Verification items for the finished model (mm, model axes). Face numbers are marked on the shaded views. A direction names the side the tool comes from. Round coordinates to 2 decimals unless told otherwise and drop trailing zeros. Order: outer loops, then holes, each group sorted by start corner. A loop starts at its lowest first (then second) coordinate and runs counter-clockwise, first axis right, second up. Notation, with made-up numbers: (51.25, -9) -> (73.25, -9) arc R21 ccw to (73.25, 5) -> close; hole circle Ø8 at (79, -30.5). An arc over 180 degrees is marked (long way). Return JSON: item names as keys, results as strings. Group by question number.
Item 1: Sectioned sample at D-D on z = 45.5. Record the cut outline in (x, y) (3 decimals), plus the area to 3 significant figures.
Item 2: Access from +Z, -Z, +X, -X, +Y, -Y to the whole of each face (thin tool, end or side, straight path). Record for the marked faces 4 and 5.
Item 3: Sectioned sample at A-A on x = 58.5. Record the cut outline in (y, z) (3 decimals), plus the area to 3 significant figures.
Item 4: Sectioned sample at C-C on y = 19. Record the cut outline in (x, z) (3 decimals).
Item 5: Sectioned sample at B-B on z = 27.5. Record the cut outline in (x, y) (3 decimals), plus the area to 3 significant figures.
Item 6: Draft check along Z on the marked faces 1, 2 and 3. Enter one of: pulls with the +Z half, pulls with the -Z half, needs draft (parallel to the pull), parting line crosses it, or undercut.
Item 7: Depth check by flat-ended pin: pin 1 Ø1 at (y, z) = (4.5, -1.5) entering from -X; pin 2 Ø1 at (y, z) = (6.5, -1) entering from +X; pin 3 Ø2 at (x, z) = (44.5, 22) entering from +Y. Enter the tip coordinate at first touch or a pass-through.
Item 8: Scan lines: probe 1 along Z at (x, y) = (33, 21) (3 decimals); probe 2 along X at (y, z) = (7.5, -1) (3 decimals); probe 3 along X at (y, z) = (34, 35.5) (3 decimals). Record each from-to range of solid material in increasing order. Write a range as from..to.
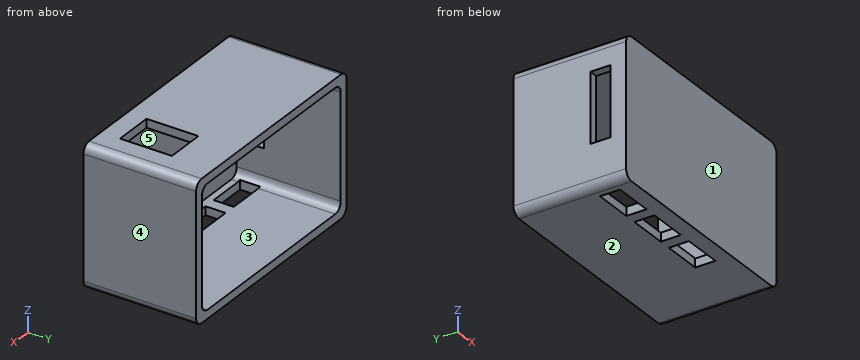
```python
from build123d import *

# Parameters (mm, degrees)
SKETCH1_W           = 76.2
SKETCH1_H           = 44.45
BOSS_EXTRUDE1_DEPTH = 38.1
SHELL1_T            = 3.175
SKETCH3_W           = 25.4
SKETCH3_H           = 7.366
CUT_EXTRUDE2_DEPTH  = 12.7
FILLET1_R           = 3.048
SKETCH6_W           = 14.605
SKETCH6_H           = 19.05
CUT_EXTRUDE4_DEPTH  = 12.7
SKETCH5_W           = 14.478
SKETCH5_H           = 7.366
CUT_EXTRUDE5_DEPTH  = 12.7


with BuildPart() as part:
    # Sketch1 → Boss-Extrude1 (new body)
    with BuildSketch(Plane(origin=(0, 0, 0), x_dir=(1, 0, 0), z_dir=(0, 1, 0))):
        with Locations((38.1, -22.225)):
            Rectangle(SKETCH1_W, SKETCH1_H)
    extrude(amount=BOSS_EXTRUDE1_DEPTH)

    # Shell1
    shell1_openings = [part.faces().sort_by_distance(p)[0] for p in [
        (38.1, 38.1, 22.225),
    ]]
    offset(amount=SHELL1_T, openings=shell1_openings, kind=Kind.INTERSECTION)

    # Sketch3 → Cut-Extrude2 (cut)
    with BuildSketch(Plane.ZY.offset(3.175)):
        with Locations((25.4, 6.223)):
            Rectangle(SKETCH3_W, SKETCH3_H)
    extrude(amount=-CUT_EXTRUDE2_DEPTH, mode=Mode.SUBTRACT)

    # Fillet1
    fillet1_edges = [part.edges().sort_by_distance(p)[0] for p in [
        (0, 19.05, 0),
        (0, 19.05, 44.45),
        (76.2, 19.05, 44.45),
        (76.2, 19.05, 0),
        (-3.175, 17.4625, -3.175),
        (79.375, 17.4625, -3.175),
        (79.375, 17.4625, 47.625),
        (-3.175, 17.4625, 47.625),
    ]]
    fillet(fillet1_edges, radius=FILLET1_R)

    # Sketch6 → Cut-Extrude4 (cut)
    with BuildSketch(Plane.XY.offset(47.625)):
        with Locations((62.5475, 13.335)):
            Rectangle(SKETCH6_W, SKETCH6_H)
    extrude(amount=-CUT_EXTRUDE4_DEPTH, mode=Mode.SUBTRACT)

    # Sketch5 → Cut-Extrude5 (cut)
    with BuildSketch(Plane(origin=(0, 0, -3.175), x_dir=(-1, 0, 0), z_dir=(0, 0, -1))):
        with Locations((-47.117, 6.223)):
            Rectangle(SKETCH5_W, SKETCH5_H)
        with Locations((-28.194, 6.223)):
            Rectangle(SKETCH5_W, SKETCH5_H)
        with Locations((-9.271, 6.223)):
            Rectangle(SKETCH5_W, SKETCH5_H)
    extrude(amount=-CUT_EXTRUDE5_DEPTH, mode=Mode.SUBTRACT)


solid = part.part
```
Recorded:
{
 "1": {"outline": "(-3.032, -3.175) -> (79.232, -3.175) -> (79.232, 38.1) -> (-3.032, 38.1) -> close; hole (55.245, 3.81) -> (69.85, 3.81) -> (69.85, 22.86) -> (55.245, 22.86) -> close", "area": "3,120 mm²"},
 "2": {"face 4": "+Z, -Z, +X, +Y, -Y", "face 5": "+Y"},
 "3": {"outline": "(-3.175, -3.175) -> (38.1, -3.175) -> (38.1, 0) -> (0, 0) -> (0, 44.45) -> (3.81, 44.45) -> (3.81, 47.625) -> (-3.175, 47.625) -> close; (22.86, 44.45) -> (38.1, 44.45) -> (38.1, 47.625) -> (22.86, 47.625) -> close", "area": "343 mm²"},
 "4": {"outline": "(-3.175, -0.127) arc R3.048 ccw to (-0.127, -3.175) -> (76.327, -3.175) arc R3.048 ccw to (79.375, -0.127) -> (79.375, 44.577) arc R3.048 ccw to (76.327, 47.625) -> (69.85, 47.625) -> (69.85, 44.45) -> (73.152, 44.45) arc R3.048 cw to (76.2, 41.402) -> (76.2, 3.048) arc R3.048 cw to (73.152, 0) -> (3.048, 0) arc R3.048 cw to (0, 3.048) -> (0, 41.402) arc R3.048 cw to (3.048, 44.45) -> (55.245, 44.45) -> (55.245, 47.625) -> (-0.127, 47.625) arc R3.048 ccw to (-3.175, 44.577) -> close"},
 "5": {"outline": "(-3.175, -3.175) -> (79.375, -3.175) -> (79.375, 38.1) -> (76.2, 38.1) -> (76.2, 0) -> (0, 0) -> (0, 2.54) -> (-3.175, 2.54) -> close; (-3.175, 9.906) -> (0, 9.906) -> (0, 38.1) -> (-3.175, 38.1) -> close", "area": "481 mm²"},
 "6": {"face 1": "needs draft", "face 2": "pulls with the -Z half", "face 3": "undercut"},
 "7": {"pin 1": "x = -3.05", "pin 2": "x = 79.35", "pin 3": "y = 0"},
 "8": {"probe 1": "-3.175..0, 44.45..47.625", "probe 2": "-3.047..2.032, 16.51..20.955, 35.433..39.878, 54.356..79.247", "probe 3": "-3.175..0, 76.2..79.375"}
}
